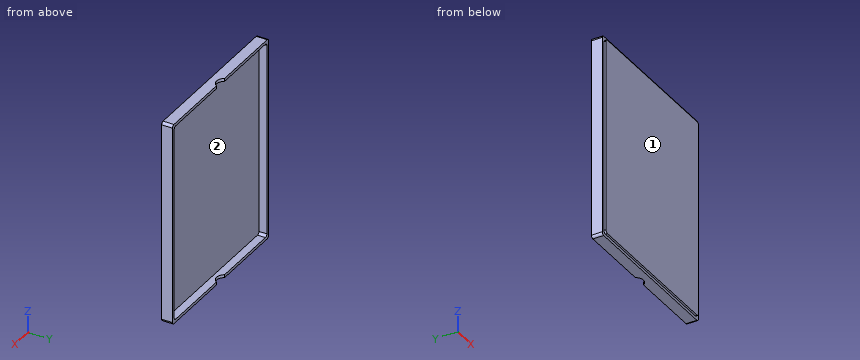
from build123d import *

# Parameters (mm, degrees)
SKETCH1_W           = 160
SKETCH1_H           = 200
BOSS_EXTRUDE1_DEPTH = 8
SHELL1_T            = 3
SKETCH2_W           = 160
SKETCH2_H           = 200
BOSS_EXTRUDE2_DEPTH = 2
FILLET1_R           = 2.5
CUT_EXTRUDE4_DEPTH  = 223.236360661


with BuildPart() as part:
    # Sketch1 → Boss-Extrude1 (new body)
    with BuildSketch(Plane(origin=(0, 0, 0), x_dir=(1, 0, 0), z_dir=(0, 1, 0))):
        Rectangle(SKETCH1_W, SKETCH1_H)
    extrude(amount=BOSS_EXTRUDE1_DEPTH)

    # Shell1
    shell1_openings = [part.faces().sort_by_distance(p)[0] for p in [
        (0, 8, 0),
    ]]
    offset(amount=SHELL1_T, openings=shell1_openings, kind=Kind.INTERSECTION)

    # Sketch2 → Boss-Extrude2 (add)
    with BuildSketch(Plane.XZ.offset(3)):
        Rectangle(SKETCH2_W, SKETCH2_H)
    extrude(amount=BOSS_EXTRUDE2_DEPTH)

    # Fillet1
    fillet1_edges = [part.edges().sort_by_distance(p)[0] for p in [
        (-80, 4, -100),
        (-80, 4, 100),
        (80, 4, 100),
        (80, 4, -100),
        (-80, -4, 100),
        (-80, -4, -100),
        (80, -4, -100),
        (80, -4, 100),
        (-83, 2.5, -103),
        (83, 2.5, -103),
        (83, 2.5, 103),
        (-83, 2.5, 103),
    ]]
    fillet(fillet1_edges, radius=FILLET1_R)

    # Sketch5 → Cut-Extrude4 (cut, through all)
    with BuildSketch(Plane.XY.offset(103)):
        with BuildLine():
            Line((0, 8), (-7, 8))
            ThreePointArc((-7, 8), (0, 4), (7, 8))
            Line((7, 8), (0, 8))
        make_face()
    extrude(amount=-CUT_EXTRUDE4_DEPTH, mode=Mode.SUBTRACT)


solid = part.part
Can you work these out from the model? Positions are in its coordinate system, mm. Face numbers are marked on the shaded views. Round coordinates to 2 decimals unless told otherwise and drop trailing zeros. Write each loop counter-clockwise with the first axis right and the second up, starting at its lowest first coordinate (ties: lowest second). Pieces come first, ordered by that corner, then holes. Notation, with made-up numbers: (62, 1) -> (118, 1) arc R34 ccw to (118, 39) -> close; hole circle Ø8 at (89.5, 59). An arc over 180 degrees is marked (long way). Use one line per item in the form item = value. Start each with the question number.
Q1. If I drill on probe 1 along X at (y, z) = (1.75, 71.5); probe 2 along Z at (x, y) = (-14, 3); probe 3 along Y at (x, z) = (34.5, 15), over which ranges is the centre line in solid material (lowest first)? Write a range as [from, to].
Q2. Imagine slicing it at B-B (x = 24). Please give me the cut outline in (y, z), then the cut area to 3 significant figures.
Q3. We'd pull the mould along X, two halves only. Please class the marked faces 1 and 2: +X half, -X half, draft (parallel to the pull), parting line (faces both ways), or undercut.
Q4. I'm going to push flat-ended pins straight in: P1, Ø6, axis at x = -35.5, z = -7.5, coming from the +Y side; P2, Ø1.6, axis at x = 34.5, y = -4, coming from the +Z side; P3, Ø1.6, axis at y = -4, z = -30, coming from the -X side. Where does each tip first touch, or does it pass through?
Q5. Imagine slicing it at A-A (z = -80). Please give me the cut outline in (x, y), then the cut area to 3 significant figures.
Worked out:
q1.probe_1 = [-83, -80], [80, 83]
q1.probe_2 = [-103, -100], [100, 103]
q1.probe_3 = [-5, 0]
q2.outline = (-5, -100) -> (-3, -100) -> (-3, -103) -> (8, -103) -> (8, -100) -> (0, -100) -> (0, 100) -> (8, 100) -> (8, 103) -> (-3, 103) -> (-3, 100) -> (-5, 100) -> close
q2.area = 1,070 mm^2
q3.face_1 = draft
q3.face_2 = undercut
q4.P1 = 0
q4.P2 = 100
q4.P3 = -80
q5.outline = (-83, -3) -> (-80, -3) -> (-80, -5) -> (80, -5) -> (80, -3) -> (83, -3) -> (83, 8) -> (80, 8) -> (80, 0) -> (-80, 0) -> (-80, 8) -> (-83, 8) -> close
q5.area = 866 mm^2
